Here's how the part is built. I have some questions about the finished solid (model axes, mm). A direction names the side the tool comes from. Coordinates: 2 decimals unless noted, no trailing zeros. Loops run counter-clockwise (first coordinate to the right, second up) from the corner with the lowest first, then second, coordinate; pieces in that order, holes last. Notation, with made-up numbers: M -7,5 L 15,5 A11 cw 15,25 Z; hole C 49.25,43 d1. An arc over 180 degrees is marked long. Use CSV: the item, a comma, the result in double quotes. Start each with the question number.
Q1. Which directions (+Z, -Z, +X, -X, +Y, -Y) give clear straight access to the entire face, cutting with the end or side of a thin tool? Please do faces 4 (the flat face through (0, -12.5, 1)), 5 (the flat face through (-26, -3, -6)), 6 (the flat face through (0, 14, 0)), 7 (the flat face through (-23, -6.5, -10)).
Q2. Please list where these lines run through material, in increasing order: probe 1 along Z at (x, y) = (23, -0.75) (3 decimals); probe 2 along X at (y, z) = (0.25, -13) (1 decimal); probe 3 along Z at (x, y) = (-23, -2.25). Write a range as [from, to].
Q3. If we section it at D-D (z = -13): Please give me the cut outline in (x, y) (1 decimal), and give its area (3 significant figures).
Q4. If we section it at A-A (y = -1): Please give me the cut outline in (x, z) (1 decimal).
Q5. If we mould it in two halves opening along X, with no side actions, what happens to faces 1 (the flat face through (26, -3, -4)), 2 (the cylindrical face through (22.145, -10.432, -0.958)), 3 (the flat face through (-23, -1, -16))? For each: +X half, -X half, draft (parallel to the pull), parting line (faces both ways), or undercut.
Q6. For pin 1 Ø4 at (x, z) = (23, -13) entering from +Y; pin 2 Ø1.8 at (x, z) = (-22.5, -7.5) entering from -Y; pin 3 Ø7 at (x, y) = (10.5, 11) entering from -Z, each with a flat end and sliding along its axis, tell me the tip position at first contact or that it passes through.
Q7. If we section it at B-B (z = -4.75): Please give me the cut outline in (x, y), and give its area (3 significant figures).
Q8. If we section it at C-C (x = 17.5): Please give me the cut outline in (y, z).
Autodesk Fusion 360 part; units mm, degrees
sketch "Sketch1" plane through (0, 0, 0) normal (0, 0, 1) x (1, 0, 0)
  line L0 (26, -17.5) -> (-26, -17.5)
  line L1 (-26, -17.5) -> (-26, 17.5)
  line L2 (-26, 17.5) -> (26, 17.5)
  line L3 (26, 17.5) -> (26, -17.5)
  line L4 (26, -17.5) -> (-26, 17.5) construction
  line L5 (-26, -17.5) -> (26, 17.5) construction
  line L6 (-20, -12.5) -> (20, -12.5)
  line L7 (20, -12.5) -> (20, 12.5)
  line L8 (20, 12.5) -> (-20, 12.5)
  line L9 (-20, 12.5) -> (-20, -12.5)
  line L10 (-20, -12.5) -> (20, 12.5) construction
  line L11 (20, -12.5) -> (-20, 12.5) construction
  dimension "d1" = 52
  dimension "d2" = 35
  dimension "d3" = 40
  dimension "d4" = 25
extrude "Extrude1" add sketch "Sketch1" along normal blind 2
sketch "Sketch2" plane through (0, 0, 0) normal (0, 0, 1) x (1, 0, 0)
sketch "Sketch3" plane through (0, 0, 0) normal (0, 0, 1) x (1, 0, 0)
  line L0 (-20, -12.5) -> (-26, -12.5)
  line L1 (-26, -12.5) -> (-26, -6.5)
  line L2 (-26, -6.5) -> (-20, -6.5)
  line L3 (-20, -6.5) -> (-20, -12.5)
  dimension "d7" = 6
extrude "Extrude2" add sketch "Sketch3" against normal blind 4
sketch "Sketch4" plane through (0, 0, 0) normal (0, 0, 1) x (1, 0, 0)
  line L0 (20, -12.5) -> (26, -12.5)
  line L1 (26, -12.5) -> (26, -6.5)
  line L2 (26, -6.5) -> (20, -6.5)
  line L3 (20, -6.5) -> (20, -12.5)
  dimension "d10" = 6
  dimension "d11" = 6
extrude "Extrude3" add sketch "Sketch4" against normal blind 4
sketch "Sketch5" plane through (0, 0, 0) normal (0, 0, 1) x (1, 0, 0)
  line L0 (20, -6.5) -> (26, -6.5)
  line L1 (26, -6.5) -> (26, 3.5)
  line L2 (26, 3.5) -> (20, 3.5)
  line L3 (20, 3.5) -> (20, -6.5)
  line L4 (-26, -6.5) -> (-20, -6.5)
  line L5 (-20, -6.5) -> (-20, 3.5)
  line L6 (-20, 3.5) -> (-26, 3.5)
  line L7 (-26, 3.5) -> (-26, -6.5)
  dimension "d14" = 6
  dimension "d15" = 10
  dimension "d16" = 6
  dimension "d17" = 10
extrude "Extrude4" add sketch "Sketch5" against normal blind 10 contours L0 L1 L2 L3
sketch "Sketch6" plane through (0, 0, 0) normal (0, 0, 1) x (1, 0, 0)
  line L0 (-26, -6.5) -> (-20, -6.5)
  line L1 (-20, -6.5) -> (-20, 3.5)
  line L2 (-20, 3.5) -> (-26, 3.5)
  line L3 (-26, 3.5) -> (-26, -6.5)
  dimension "d20" = 6
  dimension "d21" = 10
extrude "Extrude5" add sketch "Sketch6" against normal blind 10
extrude "Extrude6" add 1 faces at (22, 0.1667, -10) along direction (0, 0, -1) blind 6
extrude "Extrude7" add 1 faces at (-24, 0.1667, -10) along direction (0, 0, -1) blind 6
sketch "Sketch7" plane through (0, -6.5, 0) normal (0, -1, 0) x (1, 0, 0)
  line L0 (26, -4) -> (20, -4)
  line L1 (20, -4) -> (20, -16)
  line L2 (20, -16) -> (26, -16)
  line L3 (26, -16) -> (26, -4)
  point P0 (23, -13)
  point P1 (23, -7)
  point P2 (-23, -13)
  point P3 (-23, -7)
hole "Hole1" at (23, -6.5, -13) at (23, -6.5, -7) direction (0, 1, 0) diameter 2.93 depth 10 tip angle 118
sketch "Sketch8" plane through (0, -6.5, 0) normal (0, -1, 0) x (1, 0, 0)
  line L0 (-20, -4) -> (-26, -4)
  line L1 (-26, -4) -> (-26, -16)
  line L2 (-26, -16) -> (-20, -16)
  line L3 (-20, -16) -> (-20, -4)
  point P0 (-23, -13)
  point P1 (-23, -7)
hole "Hole2" at (-23, -6.5, -13) at (-23, -6.5, -7) direction (0, 1, 0) diameter 2.529 depth 10 tip angle 118
sketch "Sketch9" plane through (0, 0, -4) normal (0, 0, -1) x (1, 0, 0)
  line L0 (20, 12.5) -> (20, 6.5)
  line L1 (20, 6.5) -> (26, 6.5)
  line L2 (26, 6.5) -> (26, 12.5)
  line L3 (26, 12.5) -> (20, 12.5)
  point P0 (23, 9.5)
  point P1 (-23.051, 9.5)
hole "Hole3" at (-23.051, -9.5, -4) at (23, -9.5, -4) direction (0, 0, 1) diameter 2.529 depth 6 tip angle 118
Results below:
1,face 4,"+Z, -Z"
1,face 5,"+Z, -Z, -X, +Y, -Y"
1,face 6,"-Z, +X, -X, +Y"
1,face 7,"-Z, +X, -X, -Y"
2,probe 1,"[-16, -14.465], [-11.535, -8.465], [-5.535, 2]"
2,probe 2,"[-26, -24.3], [-21.7, -20], [20, 21.5], [24.5, 26]"
2,probe 3,"[-16, -14.26], [-11.74, -8.26], [-5.74, 2]"
3,outline,"M -26,-6.5 L -24.3,-6.5 L -24.3,3.5 L -26,3.5 Z; M -21.7,-6.5 L -20,-6.5 L -20,3.5 L -21.7,3.5 Z; M 20,-6.5 L 21.5,-6.5 L 21.5,3.5 L 20,3.5 Z; M 24.5,-6.5 L 26,-6.5 L 26,3.5 L 24.5,3.5 Z"
3,area,"65.4 mm^2"
4,outline,"M -26,-16 L -20,-16 L -20,2 L -26,2 Z; M 20,-16 L 26,-16 L 26,2 L 20,2 Z; hole C -23,-13 d2.5; hole C -23,-7 d2.5; hole C 23,-13 d2.9; hole C 23,-7 d2.9"
5,face 1,"+X half"
5,face 2,"undercut"
5,face 3,"draft"
6,pin 1,"y = 3.5"
6,pin 2,"y = -6.5"
6,pin 3,"z = 0"
7,outline,"M -26,-6.5 L -20,-6.5 L -20,3.5 L -26,3.5 Z; M 20,-6.5 L 26,-6.5 L 26,3.5 L 20,3.5 Z"
7,area,"120 mm^2"
8,outline,"M -17.5,0 L -12.5,0 L -12.5,2 L -17.5,2 Z; M 12.5,0 L 17.5,0 L 17.5,2 L 12.5,2 Z"
